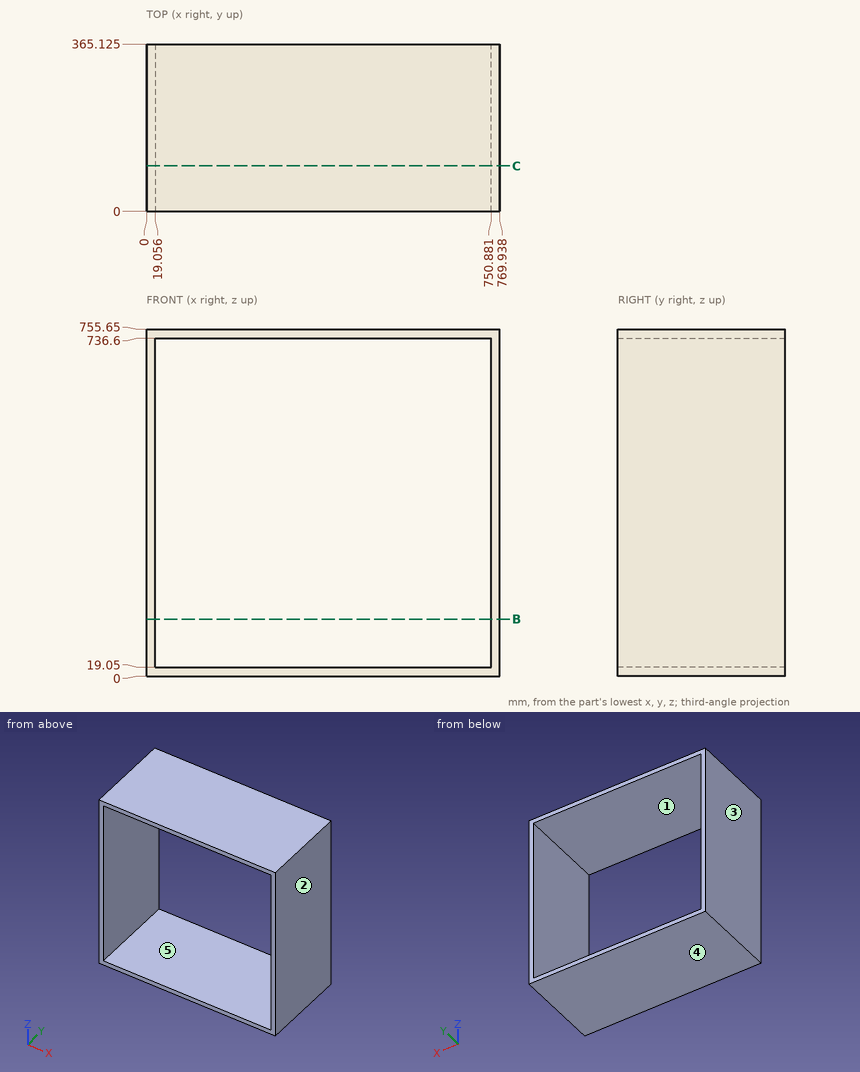
Could you check a few things on this drawing? It's one solid part, dimensions in mm from its lowest x, y, z. A direction names the side the tool comes from. Coordinates: 2 decimals unless noted, no trailing zeros. Order: outer loops, then holes, each group sorted by start corner. A loop starts at its lowest first (then second) coordinate and runs counter-clockwise, first axis right, second up. Notation, with made-up numbers: M -25.5,9.25 L 29.5,9.25 A20 ccw 29.5,25.25 Z; hole C 26,-17.75 d3. An arc over 180 degrees is marked long. Answer as a JSON object with one key per item and string values. Group by question number.
(1) Suppose I cut it at B-B, the plane z = 124. Please give me the cut outline in (x, y) (1 decimal).
(2) Suppose I cut it at C-C, the plane y = 99.5. Please give me the cut outline in (x, z), then the cut area to 3 significant figures.
(3) For pin 1 (8 mm diameter, centred on y = 314, z = 90.5, fed in from -X), with a flat end and sliding along its axis, tell me the tip position at first contact or that it passes through.
(4) I need wall thicknesses on probe 1 along Z at (x, y) = (103, 335.5); probe 2 along X at (y, z) = (228, 288). Which ranges of each line are inside material? Lowest first, please.
(5) If we mould it in two halves opening along X, with no side actions, what happens to the marked faces 1, 2 and 3? For each: released by +X, released by -X, zero draft, split by the parting line, or undercut.
(6) Which directions (+Z, -Z, +X, -X, +Y, -Y) give clear straight access to the entire face, cutting with the end or side of a thin tool? Please do the marked faces 4 and 5.
Values found:
{
 "1": {"outline": "M 0,0 L 19.1,0 L 19.1,365.1 L 0,365.1 Z; M 750.9,0 L 769.9,0 L 769.9,365.1 L 750.9,365.1 Z"},
 "2": {"outline": "M 0,0 L 769.94,0 L 769.94,755.65 L 0,755.65 Z; hole M 19.06,19.05 L 750.88,19.05 L 750.88,736.6 L 19.06,736.6 Z", "area": "56,700 mm^2"},
 "3": {"pin 1": "stops at x = 0"},
 "4": {"probe 1": "z = 0 to 19.05, 736.6 to 755.65", "probe 2": "x = 0 to 19.06, 750.88 to 769.94"},
 "5": {"face 1": "undercut", "face 2": "released by +X", "face 3": "released by -X"},
 "6": {"face 4": "-Z, +X, -X, +Y, -Y", "face 5": "+Y, -Y"}
}
